from build123d import *

# Parameters (mm, degrees)
F0_W     = 914.4
F0_H     = 955.675
F2_DEPTH = 9.525
F1_W     = 904.875
F1_H     = 895.35
F1_H_2   = 31.75
F3_DEPTH = 9.525
F5_D     = 6.35
F5_DEPTH = 6.35
F5_TIP   = 1.9077324654


with BuildPart() as f2:
    # F0 (on Right) → F2 (new body)
    with BuildSketch(Plane.YZ):
        Rectangle(F0_W, F0_H)
    extrude(amount=F2_DEPTH)

    # F1 (on face) → F3 (join)
    with BuildSketch(Plane.YZ):
        with Locations((-4.7625, 20.6375)):
            Rectangle(F1_W, F1_H)
        with Locations((-4.7625, -461.9625)):
            Rectangle(F1_W, F1_H_2)
    extrude(amount=-F3_DEPTH)

    # F5
    with Locations(Plane(origin=(-9.525, 0, 0), x_dir=(0, -1, 0), z_dir=(-1, 0, 0))):
        with Locations((-355.6, 274.6375), (355.6, -233.3625), (-355.6, -30.1625), (355.6, 71.4375), (355.6, -30.1625), (0, -30.1625), (0, -233.3625), (355.6, 274.6375), (0, -131.7625), (0, 71.4375), (-355.6, 71.4375), (-355.6, -131.7625), (0, 274.6375), (-355.6, 173.0375), (355.6, 173.0375), (0, 173.0375), (355.6, -131.7625), (-355.6, -233.3625)):
            Hole(F5_D / 2, depth=F5_DEPTH)
            with Locations((0, 0, -(F5_DEPTH + F5_TIP / 2))):  # 118° drill point
                Cone(0, F5_D / 2, F5_TIP, mode=Mode.SUBTRACT)


solid = f2.part
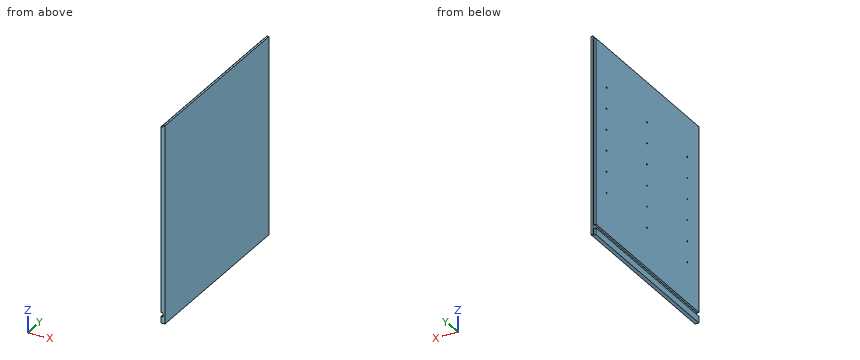
Check sheet for the modelled part. Datum: model origin and axes. Units: mm. Round coordinates to 2 decimals unless told otherwise and drop trailing zeros. One line per item, written item: value.
(1) Depth check by flat-ended pin: pin 1 Ø5 at (x, z) = (-5, -23) entering from +Y (3 decimals); pin 2 Ø3 at (x, y) = (-5, 182.5) entering from +Z; pin 3 Ø5 at (y, z) = (355.6, 71.44) entering from -X. Enter the tip coordinate at first touch or a pass-through.
Computed values:
pin 1: stops at y = 447.675
pin 2: stops at z = 468.31
pin 3: stops at x = -2.77
(2) Thickness scan on line 1 (Y direction, x = -3.5, z = 175) (3 decimals); line 2 (Z direction, x = -6, y = -294.5); line 3 (Y direction, x = -4, z = -6) (3 decimals). Record the ranges inside material, lowest first.
Computed values:
line 1: y = -457.2 to -358.096, -353.104 to -2.496, 2.496 to 353.104, 358.096 to 447.675
line 2: z = -477.84 to -446.09, -427.04 to 468.31
line 3: y = -457.2 to 447.675
(3) Sectioned sample at A-A, the plane x = -6.5. Count the separate pieces of the cut face and the enclosed holes in it, then the cut area to 3 significant figures.
Computed values:
separate pieces: 2
enclosed holes: 18
area: 838,000 mm^2
